Could you check a few things on this model? Use its own coordinates, in mm. A direction names the side the tool comes from. Round coordinates to 2 decimals unless told otherwise and drop trailing zeros. Write each loop counter-clockwise with the first axis right and the second up, starting at its lowest first coordinate (ties: lowest second). Pieces come first, ordered by that corner, then holes. Notation, with made-up numbers: (-7.75, -33.5) -> (19.25, -33.5) arc R10 ccw to (19.25, -15.5) -> close; hole circle Ø11 at (47, 70.5). An arc over 180 degrees is marked (long way). Answer in a Markdown table with one row per item. Add a question column.
```python
from build123d import *

# Parameters (mm, degrees)
F0_W      = 25.4
F0_H      = 76.2
F1_DEPTH  = 1
F3_DEPTH  = 1
F8_R      = 2.54
F9_DEPTH  = 1.0010001
F11_DEPTH = 1.0010001


with BuildPart() as f1:
    # F0 (on Top) → F1 (new body)
    with BuildSketch(Plane.XY):
        Rectangle(F0_W, F0_H)
        Polygon((-6.35, -31.75), (-6.35, 31.75), (-3.81, 31.75), (3.81, 31.75), (6.35, 31.75), (6.35, -31.75), align=None, mode=Mode.SUBTRACT)
        Polygon((3.81, 31.75), (-3.81, 31.75), (-3.81, 29.21), (-3.81, -29.21), (3.81, -29.21), (3.81, 29.21), align=None)
    extrude(amount=F1_DEPTH)

    # F2 (on Top) → F3 (join)
    with BuildSketch(Plane.XY):
        with BuildLine():
            ThreePointArc((12.7, 42.9509683429), (17.3901912008, 49.3728700667), (19.05, 57.15))
            ThreePointArc((19.05, 57.15), (0, 76.2), (-19.05, 57.15))
            ThreePointArc((-19.05, 57.15), (-17.3901912008, 49.3728700667), (-12.7, 42.9509683429))
            ThreePointArc((-12.7, 42.9509683429), (0, 38.1), (12.7, 42.9509683429))
        make_face()
        with BuildLine():
            Line((12.7, 33.2490316571), (12.7, 42.9509683429))
            ThreePointArc((12.7, 42.9509683429), (0, 38.1), (-12.7, 42.9509683429))
            Line((-12.7, 42.9509683429), (-12.7, 33.2490316571))
            Line((-12.7, 33.2490316571), (12.7, 33.2490316571))
        make_face()
    extrude(amount=F3_DEPTH)

    # F7: sweep along a path in F6
    with BuildLine(Plane.XY.offset(1)) as f7_path:
        CenterArc((0, 57.15), 19.05, 0, 360)
    # F5 (on offset) → F7 (sweep)
    with BuildSketch(Plane.XZ.offset(-57.15)):
        with BuildLine():
            Line((-19.05, 0), (-15.6564548698, 0))
            ThreePointArc((-15.6564548698, 0), (-17.3532274349, 2.3092691054), (-19.05, 0))
        make_face()
    sweep(path=f7_path.line)

    # F8 (on face) → F9 (cut, through all)
    with BuildSketch(Plane.XY.offset(1)):
        with Locations((-6.35, 63.5)):
            Circle(F8_R)
        with Locations((6.35, 63.5)):
            Circle(F8_R)
    extrude(amount=-F9_DEPTH, mode=Mode.SUBTRACT)

    # F10 (on face) → F11 (cut, through all)
    with BuildSketch(Plane.XY.offset(1)):
        with BuildLine():
            ThreePointArc((10.16, 57.15), (0, 51.4801930411), (-10.16, 57.15))
            ThreePointArc((-10.16, 57.15), (0, 46.99), (10.16, 57.15))
        make_face()
    extrude(amount=-F11_DEPTH, mode=Mode.SUBTRACT)


solid = f1.part
```
(1) If we mould it in two halves opening along X, with no side actions, what happens to faces 1 (the face through (0, 33, 0)), 2 (the face through (-6.9, 61.02, 0.51))? For each: pulls with the +X half, pulls with the -X half, needs draft (parallel to the pull), parting line crosses it, or undercut.
(2) Suppose I cut it at D-D, the plane z = 1.7. Please give me the cut outline in (x, y), then the cut area to 3 significant figures.
(3) Suppose I cut it at A-A, the plane y = -11. Please give me the cut outline in (x, z).
(4) Suppose I cut it at B-B, the plane x = 0. Please give me the cut outline in (y, z), then the cut area to 3 significant figures.
(5) On a 3-axis mill with a long thin cutter (end or side, diameter ignored), from which of +Z, -Z, +X, -X, +Y, -Y can I reach the whole of each face in a straight line? I mean faces 3 (the face through (5.8, 61.02, 0.51)), 4 (the face through (0, 57, 1)). Say none if no direction works.
(6) For P1, Ø1.1, axis at y = 9.5, z = 0.5, coming from the +X side; P2, Ø6, axis at x = 6.35, y = 63.5, coming from the +Z side; P3, Ø1.1, axis at x = -0.5, z = 0.5, coming from the +Y side, each with a flat end and sliding along its axis, tell me the tip position at first contact or that it passes through.
(7) I need wall thicknesses on L1, parallel to X at y = 1, z = 0.3; L2, parallel to Y at x = 8, z = 0.95; L3, parallel to X at y = 57, z = 1.1. Which ranges of each line are inside material? Lowest first, please.
(8) Suppose I cut it at C-C, the plane y = -30.5. Please give me the cut outline in (x, z).
Response:
| question | item | result |
|---|---|---|
| 1 | face 1 | needs draft |
| 1 | face 2 | undercut |
| 2 | outline | circle Ø37.39 at (0, 57.15); hole circle Ø32.03 at (0, 57.15) |
| 2 | area | 292 mm² |
| 3 | outline | (-12.7, 0) -> (-6.35, 0) -> (-6.35, 1) -> (-12.7, 1) -> close; (-3.81, 0) -> (3.81, 0) -> (3.81, 1) -> (-3.81, 1) -> close; (6.35, 0) -> (12.7, 0) -> (12.7, 1) -> (6.35, 1) -> close |
| 4 | outline | (-38.1, 0) -> (-31.75, 0) -> (-31.75, 1) -> (-38.1, 1) -> close; (-29.21, 0) -> (46.99, 0) -> (46.99, 1) -> (41.51, 1) arc R1.78 ccw to (38.08, 1) -> (-29.21, 1) -> close; (51.48, 0) -> (76.2, 0) arc R1.78 ccw (long way) to (72.79, 1) -> (51.48, 1) -> close |
| 4 | area | 114 mm² |
| 5 | face 3 | +Z, -Z |
| 5 | face 4 | +Z |
| 6 | P1 | x = 12.7 |
| 6 | P2 | z = 1 |
| 6 | P3 | y = 76.28 |
| 7 | L1 | -12.7 to -6.35, -3.81 to 3.81, 6.35 to 12.7 |
| 7 | L2 | -38.1 to 50.89, 54.56 to 61.57, 65.43 to 74.47 |
| 7 | L3 | -19.04 to -15.67, 15.67 to 19.04 |
| 8 | outline | (-12.7, 0) -> (-6.35, 0) -> (-6.35, 1) -> (-12.7, 1) -> close; (6.35, 0) -> (12.7, 0) -> (12.7, 1) -> (6.35, 1) -> close |
